Design review of the part shown in the three views and the two pictorial views. Dimensions are in mm from the part's minimum x, y and z. A direction names the side the tool comes from. Round coordinates to 2 decimals unless told otherwise and drop trailing zeros. Loops run counter-clockwise (first coordinate to the right, second up) from the corner with the lowest first, then second, coordinate; pieces in that order, holes last. Notation, with made-up numbers: (-28, 34) -> (13, 34) arc R4 cw to (13, 39) -> close; hole circle Ø11 at (-21, -31). An arc over 180 degrees is marked (long way). Use CSV: the item, a comma, the result in double quotes. Start each with the question number.
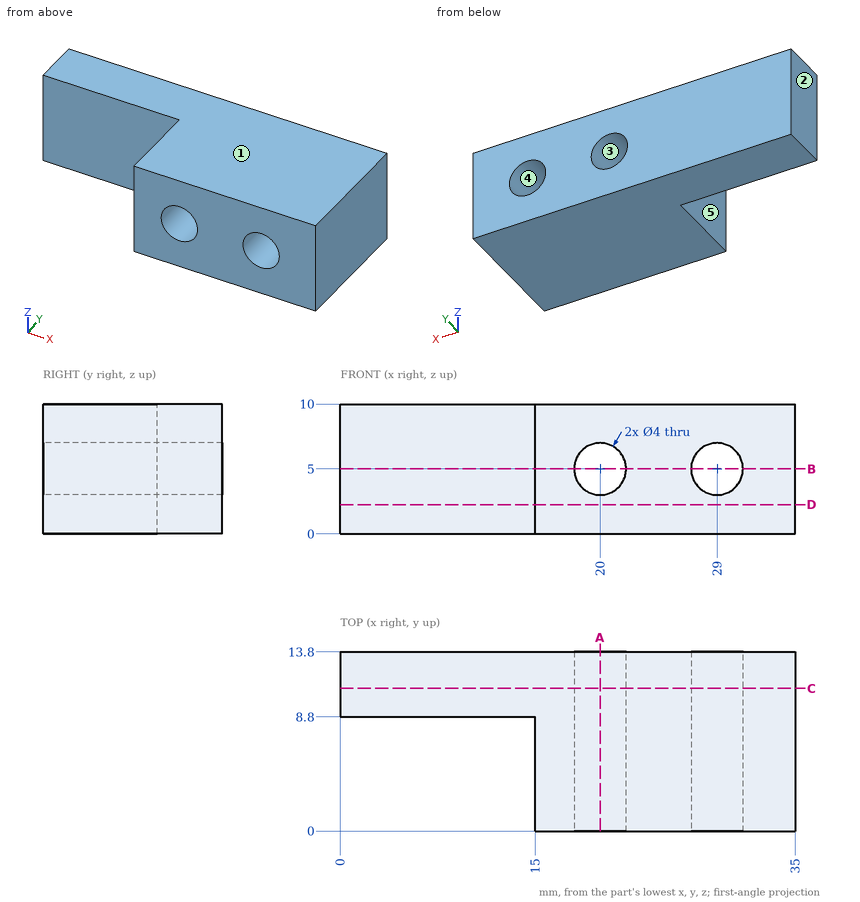
1. For line 1 along X through (y, z) = (1.25, 4); line 2 along Z through (x, y) = (29, 7.75); line 3 along Y through (x, z) = (8.5, 3.5), list the stretches that pass through material, from the lowest coordinate up. Write a range as from..to.
2. Take a section at A-A, the plane x = 20. Give the boundary of the cut face in (y, z), then the cut area to 3 significant figures.
3. The part is to be moulded in two halves that separate along Z. For the marked faces 1, 2 and 3, say which applies: pulls with the +Z half, pulls with the -Z half, needs draft (parallel to the pull), parting line crosses it, or undercut.
4. For the marked faces 4 and 5, list the 3-axis set-ups (+Z, -Z, +X, -X, +Y, -Y) from which the entire face can be reached by the end or side of a thin tool; tool diameter is ignored.
5. Take a section at C-C, the plane y = 11. Give the boundary of the cut face in (x, z).
6. Take a section at B-B, the plane z = 5. Give the boundary of the cut face in (x, y), then the cut area to 3 significant figures.
7. Take a section at D-D, the plane z = 2.25. Give the boundary of the cut face in (x, y), then the cut area to 3 significant figures.
8. Clearance check with flat-ended pins moving along their axes: P1, Ø5, axis at x = 4.5, z = 3, coming from the -Y side; P2, Ø4.5, axis at y = 4.5, z = 6, coming from the -X side; P3, Ø3, axis at x = 20, z = 7.5, coming from the -Y side. State where each tip first meets the part, or that it passes through.
Results:
1,line 1,"15..18.27, 21.73..27.27, 30.73..35"
1,line 2,"0..3, 7..10"
1,line 3,"8.8..13.8"
2,outline,"(0, 0) -> (13.8, 0) -> (13.8, 3) -> (0, 3) -> close; (0, 7) -> (13.8, 7) -> (13.8, 10) -> (0, 10) -> close"
2,area,"82.8 mm²"
3,face 1,"pulls with the +Z half"
3,face 2,"needs draft"
3,face 3,"undercut"
4,face 4,"+Y, -Y"
4,face 5,"+Z, -Z, -X, -Y"
5,outline,"(0, 0) -> (35, 0) -> (35, 10) -> (0, 10) -> close; hole circle Ø4 at (20, 5); hole circle Ø4 at (29, 5)"
6,outline,"(0, 8.8) -> (15, 8.8) -> (15, 0) -> (18, 0) -> (18, 13.8) -> (0, 13.8) -> close; (22, 0) -> (27, 0) -> (27, 13.8) -> (22, 13.8) -> close; (31, 0) -> (35, 0) -> (35, 13.8) -> (31, 13.8) -> close"
6,area,"241 mm²"
7,outline,"(0, 8.8) -> (15, 8.8) -> (15, 0) -> (35, 0) -> (35, 13.8) -> (0, 13.8) -> close"
7,area,"351 mm²"
8,P1,"y = 8.8"
8,P2,"x = 15"
8,P3,"y = 0"
